Read the model definition and answer for the solid it produces. Units are mm, in the model's axes. Face numbers are marked on the shaded views. A direction names the side the tool comes from. Coordinates: 2 decimals unless noted, no trailing zeros. Write each loop counter-clockwise with the first axis right and the second up, starting at its lowest first coordinate (ties: lowest second). Pieces come first, ordered by that corner, then holes. Notation, with made-up numbers: (82.25, 25) - (107.25, 25) arc R23 cw to (107.25, 45) - close; hole circle Ø3 at (47, -15). An arc over 180 degrees is marked (long way). Return JSON: item names as keys, results as strings.
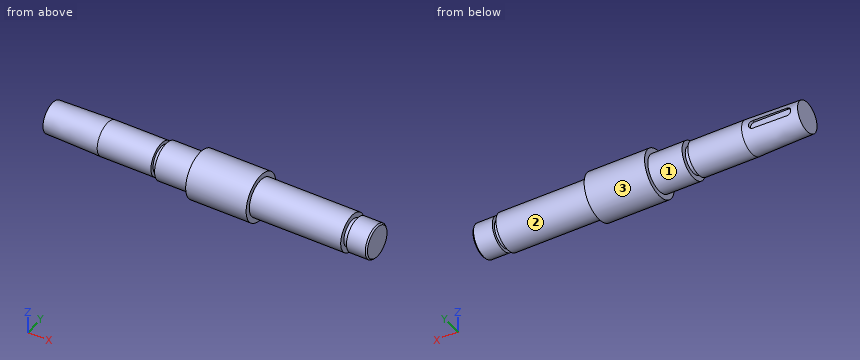
Autodesk Inventor part; units mm, degrees
ref_plane "РабПлоскость1" through (0, 25, 0) normal (0, 1, 0) x (-1, 0, 0)
ref_plane "Начальная плоскость" through (0, 0, 0) normal (1, 0, 0) x (0, 1, 0)
ref_plane "XY Plane" through (0, 0, 0) normal (0, 0, 1) x (1, 0, 0)
sketch "Основной эскиз" plane through (0, 0, 0) normal (0, 0, 1) x (1, 0, 0)
  line L0 (0, 0) -> (483, 0)
  line L1 (0, 0) -> (0, 22.95)
  line L2 (0, 22.95) -> (82, 25)
  line L3 (162, 25) -> (162, 20)
  line L4 (82, 25) -> (162, 25)
  line L5 (162, 20) -> (169, 20)
  line L6 (169, 20) -> (169, 27.5)
  line L7 (169, 27.5) -> (220, 27.5)
  line L8 (220, 27.5) -> (220, 35)
  line L9 (310, 35) -> (310, 27.5)
  line L10 (220, 35) -> (310, 35)
  line L11 (446, 27.5) -> (446, 20)
  line L12 (310, 27.5) -> (446, 27.5)
  line L13 (446, 20) -> (453, 20)
  line L14 (453, 20) -> (453, 25)
  line L15 (483, 25) -> (483, 0)
  line L16 (453, 25) -> (483, 25)
  dimension "d3" = 50
  dimension "d4" = 40
  dimension "d5" = 55
  dimension "d6" = 70
  dimension "d7" = 55
  dimension "d8" = 40
  dimension "d9" = 50
revolve "Вращение1" add sketch "Основной эскиз" angle 360 about axis through (0, 0, 0) along (1, 0, 0)
chamfer "Фаска1" distance 2 angle 45 1 edges at (483, -25, 0) measured on face at (463, 24.6763, -4.0103)
ref_plane "РабПлоскость1" through (0, 25, 0) normal (0, 1, 0) x (-1, 0, 0)
sketch "Эскиз3" plane through (0, 25, 0) normal (0, 1, 0) x (-1, 0, 0)
  line L0 (-16, 0) -> (-66, 0) construction
  line L1 (-16, 6) -> (-66, 6)
  line L2 (-66, -6) -> (-16, -6)
  arc A0 (-16, -6) -> (-16, 6) centre (-16, 0) ccw
  arc A1 (-66, 6) -> (-66, -6) centre (-66, 0) ccw
  line L3 (0, -22.95) -> (0, 22.95)
  line L4 (14.4, 0) -> (-86.4, 0)
  point P0 (0, 0)
  point P1 (-41, 0)
  dimension "d15" = 25
  dimension "d16" = 12
  dimension "d17" = 41
extrude "Выдавливание1" cut sketch "Эскиз3" against normal blind 5
equation "\"Length\" = 483"
properties part number "Вал" material "Сталь, углеродистая"
(1) Straight lines are drawn through the part: line 1 (Z direction, x = 444, y = -1); line 2 (X direction, y = -18.5, z = 17.5); line 3 (X direction, y = -22.5, z = 19). For each, find the intervals that lie inside material, in ascending order. Write a range as from..to.
Answer:
{"line 1": "-27.48..27.48", "line 2": "169..446", "line 3": "220..310"}
(2) Which of the six approach directions +Z, -Z, +X, -X, +Y, -Y give full straight-line access (tool end or side, diameter ignored) to the marked faces 1, 2 and 3?
Answer:
{"face 1": "-X", "face 2": "+X", "face 3": "+X, -X"}
(3) Flat-ended cylindrical pins translate along their axes: P1, Ø1.2, axis at x = 43, y = 22, coming from the -Z side; P2, Ø4, axis at x = 196.5, y = 3.5, coming from the -Z side; P3, Ø2, axis at y = -10, z = -27.5, coming from the +X side. Find the tip coordinate at first contact, or state that the pin passes through.
Answer:
{"P1": "z = -10.92", "P2": "z = -27.46", "P3": "x = 310"}
(4) A cutting plane is placed at B-B (x = 264). Determine the outline of the cut face in (y, z), and give its area (3 significant figures).
Answer:
{"outline": "circle Ø70 at (0, 0)", "area": "3,850 mm²"}
(5) A cutting plane is placed at C-C (x = 121). Determine the outline of the cut face in (y, z), and give its area (3 significant figures).
Answer:
{"outline": "circle Ø50 at (0, 0)", "area": "1,960 mm²"}
